Design review of the part built by this model. Coordinates are the model's own, in mm. A direction names the side the tool comes from. Round coordinates to 2 decimals unless told otherwise and drop trailing zeros. Loops run counter-clockwise (first coordinate to the right, second up) from the corner with the lowest first, then second, coordinate; pieces in that order, holes last. Notation, with made-up numbers: M 52,87.5 L 56,87.5 A23 cw 56,102.5 Z; hole C 40.5,39.25 d3. An arc over 180 degrees is marked long. Use a Markdown table: item, result.
from build123d import *

# Parameters (mm, degrees)
F0_R      = 1.7245608891
F1_DEPTH  = 3.81
F2_R      = 5.0827847808
F3_DEPTH  = 1.8796
F5_DEPTH  = 1.8034
F5_FACE_R = 5.0827847808
F4_R      = 4.0761496426
F1_FACE_R = 1.7245608891
F6_DEPTH  = 0.2032
F7_DEPTH  = 40.64


with BuildPart() as f1:
    # F0 (on Front) → F1 (new body)
    with BuildSketch(Plane.XZ):
        with BuildLine():
            ThreePointArc((-40.6846019076, 33.996454664), (-43.8586035919, 26.4801119862), (-51.985972327, 25.7620789885))
            ThreePointArc((-51.985972327, 25.7620789885), (-43.4988667945, 12.1772585573), (-28.5669643091, 17.975240502))
            ThreePointArc((-28.5669643091, 17.975240502), (-35.5078844362, 23.842234183), (-33.4709389841, 32.6993691762))
            ThreePointArc((-33.4709389841, 32.6993691762), (-36.5719585653, 36.1609542707), (-40.6846019076, 33.996454664))
        make_face()
        with Locations((-37.240639329, 32.4421264231)):
            Circle(F0_R, mode=Mode.SUBTRACT)
    extrude(amount=F1_DEPTH)

    # F2 (on Front) → F3 (join)
    with BuildSketch(Plane.XZ):
        with Locations((-41.6127927601, 19.4445531815)):
            Circle(F2_R)
    extrude(amount=-F3_DEPTH)

    # F5 (add): a face of the model
    f5_faces = [f1.faces().sort_by_distance(p)[0] for p in [
        (-41.6127927601, 1.8796, 19.4445531815),
    ]]
    extrude(f5_faces, amount=F5_DEPTH)

    # F5_face (on face) + F4 (on Front) + F1_face (on face) → F6 (join)
    with BuildSketch(Plane(origin=(-41.6127927601, 3.683, 19.4445531815), x_dir=(-1, 0, 0), z_dir=(0, 1, 0))):
        Circle(F5_FACE_R)
    with BuildSketch(Plane.XZ):
        with Locations((-41.713938117, 19.8042206466)):
            Circle(F4_R)
    with BuildSketch(Plane(origin=(-40.7069598519, -3.81, 21.1441009412), x_dir=(1, 0, 0), z_dir=(0, -1, 0))):
        with BuildLine():
            ThreePointArc((7.2360208677, 11.555268235), (4.1350012866, 15.0168533295), (0.0223579443, 12.8523537228))
            ThreePointArc((0.0223579443, 12.8523537228), (-3.15164374, 5.336011045), (-11.2790124751, 4.6179780473))
            ThreePointArc((-11.2790124751, 4.6179780473), (-2.7919069426, -8.9668423839), (12.1399955428, -3.1688604391))
            ThreePointArc((12.1399955428, -3.1688604391), (5.1990754157, 2.6981332418), (7.2360208677, 11.555268235))
        make_face()
        with Locations((3.4663205229, 11.2980254819)):
            Circle(F1_FACE_R, mode=Mode.SUBTRACT)
    extrude(amount=F6_DEPTH, dir=(0, 1, 0))

    # F7 (add): a face of the model
    f7_faces = [f1.faces().sort_by_distance(p)[0] for p in [
        (-41.6127927601, 3.8862, 19.4445531815),
    ]]
    extrude(f7_faces, amount=F7_DEPTH)


solid = f1.part
1. Take a section at B-B on z = 20.25. Give the boundary of the cut face in (x, y).
Check values:
| item | result |
|---|---|
| outline | M -51.49,-3.81 L -33.21,-3.81 L -33.21,0 L -36.59,0 L -36.59,44.53 L -46.63,44.53 L -46.63,0 L -51.49,0 Z |
2. Take a section at A-A on x = -37.5. Give the boundary of the cut face in (y, z).
Check values:
| item | result |
|---|---|
| outline | M -3.81,11.7 L 0,11.7 L 0,16.46 L 44.53,16.46 L 44.53,22.43 L 0,22.43 L 0,30.74 L -3.81,30.74 Z; M -3.81,34.15 L 0,34.15 L 0,36.21 L -3.81,36.21 Z |
3. Insertion check: pin 1 (5 mm diameter, centred on y = 5.5, z = 17.5, fed in from -X); pin 2 (1.5 mm diameter, centred on y = 31, z = 15, fed in from -X); pin 3 (4 mm diameter, centred on x = -32, z = 14.5, fed in from +Y). Each pin has a flat end and moves straight along its axis. Give the tip position at first contact, or say it passes through.
Check values:
| item | result |
|---|---|
| pin 1 | stops at x = -46.7 |
| pin 2 | stops at x = -45.1 |
| pin 3 | stops at y = 0 |
4. Wall thickness on line 1 along Y through (x, z) = (-37, 21.75); line 2 along Z through (x, y) = (-45.75, 39.5); line 3 along X through (y, z) = (3.5, 19.75): over which ranges is each line inside the solid? List them lowest first. Write a range as from..to.
Check values:
| item | result |
|---|---|
| line 1 | y = -3.81..0 |
| line 2 | z = 16.49..22.4 |
| line 3 | x = -46.69..-36.54 |
5. Take a section at C-C on x = -44.75. Give the boundary of the cut face in (y, z).
Check values:
| item | result |
|---|---|
| outline | M -3.81,12.67 L 0,12.67 L 0,15.45 L 44.53,15.45 L 44.53,23.44 L 0,23.44 L 0,25.92 L -3.81,25.92 Z |
6. Machinability: for faces 1 (the face through (-40, -3.81, 21)), 2 (the face through (-40, 0, 25)), which of the approach directions +Z, -Z, +X, -X, +Y, -Y give a long, thin tool a straight path to every point of the face, cutting with its end or side? Answer none if there is none.
Check values:
| item | result |
|---|---|
| face 1 | +Z, -Z, +X, -X, -Y |
| face 2 | +Y |
7. Take a section at D-D on y = 15. Give the boundary of the cut face in (x, z), and give its area (3 significant figures).
Check values:
| item | result |
|---|---|
| outline | C -41.61,19.44 d10.17 |
| area | 81.2 mm² |
